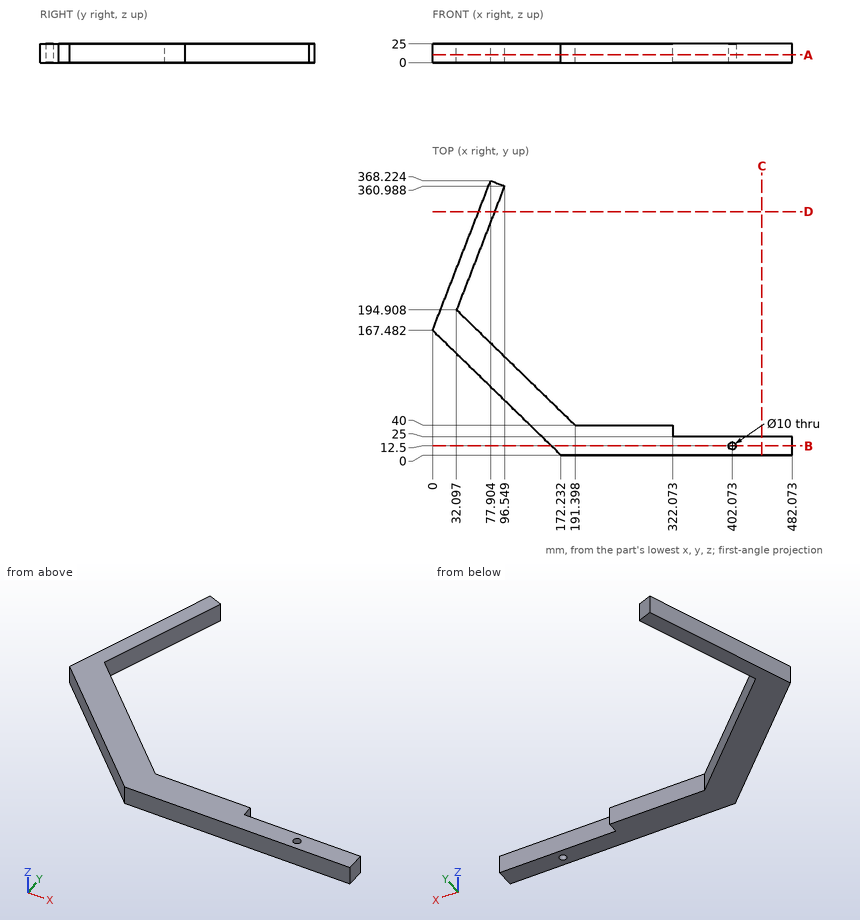
Input: dimensioned drawing with shaded views. Units: mm. Origin: part minimum x, y, z. Coordinates: 2 decimals unless noted, no trailing zeros. Loops run counter-clockwise (first coordinate to the right, second up) from the corner with the lowest first, then second, coordinate; pieces in that order, holes last. Notation, with made-up numbers: (84.25, 21) -> (98.25, 21) arc R17 cw to (98.25, 36) -> close; hole circle Ø3 at (38.25, -18.75). An arc over 180 degrees is marked (long way). Use a Markdown table: item, result. Add a question column.
(1) Section query C-C, the plane x = 441.5. Return loops of the section in (y, z), plus the area to 3 significant figures.
(2) Line query: line 1 along Y through (x, z) = (353.5, 4.25); line 2 along Y through (x, z) = (197, 15.5); line 3 along X through (y, z) = (273, 15.5). Output: solid intervals per line, ascending.
(3) Section query B-B, the plane y = 12.5. Return loops of the section in (x, z), plus the area to 3 significant figures.
(4) Pin query (flat end, axial travel): pin 1 Ø1 at (y, z) = (166.5, 15.5) entering from -X (1 decimal); pin 2 Ø7.5 at (x, z) = (224.5, 10.5) entering from +Y; pin 3 Ø8 at (y, z) = (269.5, 10) entering from +X. Return the tip coordinate at first contact, or that it passes through.
(5) Section query A-A, the plane z = 10.25. Return loops of the section in (x, y).
(6) Section query D-D, the plane y = 326.5. Return loops of the section in (x, z) (1 decimal).
Answer:
| question | item | result |
|---|---|---|
| 1 | outline | (0, 0) -> (25, 0) -> (25, 25) -> (0, 25) -> close |
| 1 | area | 625 mm^2 |
| 2 | line 1 | y = 0 to 25 |
| 2 | line 2 | y = 0 to 40 |
| 2 | line 3 | x = 40.95 to 62.4 |
| 3 | outline | (159.38, 0) -> (397.07, 0) -> (397.07, 25) -> (159.38, 25) -> close; (407.07, 0) -> (482.07, 0) -> (482.07, 25) -> (407.07, 25) -> close |
| 3 | area | 7,820 mm^2 |
| 4 | pin 1 | stops at x = 0.5 |
| 4 | pin 2 | stops at y = 40 |
| 4 | pin 3 | stops at x = 62.6 |
| 5 | outline | (0, 167.48) -> (172.23, 0) -> (482.07, 0) -> (482.07, 25) -> (322.07, 25) -> (322.07, 40) -> (191.4, 40) -> (32.1, 194.91) -> (96.55, 360.99) -> (77.9, 368.22) -> close; hole circle Ø10 at (402.07, 12.5) |
| 6 | outline | (61.7, 0) -> (83.2, 0) -> (83.2, 25) -> (61.7, 25) -> close |
